Read the model definition and answer for the solid it produces. Units are mm, in the model's axes. Face numbers are marked on the shaded views. Give positions to 0.01 mm unless a question says otherwise; leave off trailing zeros. Order: outer loops, then holes, each group sorted by start corner. A loop starts at its lowest first (then second) coordinate and runs counter-clockwise, first axis right, second up. Notation, with made-up numbers: (-14, -30) - (6, -30) arc R29 ccw to (6, 4) - close; hole circle Ø3 at (-18, 33.25). An arc over 180 degrees is marked (long way). Use a Markdown table: item, result. Add a question column.
1. A cutting plane is placed at B-B on x = 0. Determine the outline of the cut face in (y, z).
2. A cutting plane is placed at D-D on y = -2. Determine the outline of the cut face in (x, z) (1 decimal), and give its area (3 significant figures).
3. A cutting plane is placed at A-A on z = 0. Determine the outline of the cut face in (x, y).
4. Consider L1, parallel to X at y = -2.9, z = 0; L2, parallel to X at y = -4.95, z = 0; L3, parallel to Z at x = 0, y = -5.2. Determine where each line is inside the solid, lowest interval first.
5. A cutting plane is placed at C-C on y = 4. Determine the outline of the cut face in (x, z).
6. For a pull along X with two mould halves and no side action, classify the marked faces 1 and 2 as released by +X, released by -X, zero draft, split by the parting line, or undercut.
7. Flat-ended cylindrical pins translate along their axes: P1, Ø2, axis at y = 8.5, z = -7, coming from the -X side; P2, Ø1.5, axis at y = 10.5, z = -6, coming from the -X side; P3, Ø5, axis at x = 4, z = 0, coming from the +Y side; P4, Ø10, axis at x = -1.5, z = 0.5, coming from the +Y side. Find the tip coordinate at first contact, or state that the pin passes through.
```python
from build123d import *

# Parameters (mm, degrees)
TRUNCATED_BALL_DEPTH      = 13.7
TRUNCATED_BALL_DEPTH_BACK = 13.7
SKETCH8_W                 = 1.5875
SKETCH8_H                 = 11.1125


with BuildPart() as part:
    # Sketch1 → Complete_Ball (revolve)
    with BuildSketch(Plane.XY):
        with BuildLine():
            Line((0, 12.7), (0, -12.7))
            ThreePointArc((0, -12.7), (12.7, 0), (0, 12.7))
        make_face()
    revolve(axis=Axis((0, 13.6525, 0), (0, -1, 0)))

    # Sketch2 → Truncated_ball (cut, two sides)
    with BuildSketch(Plane.XY) as truncated_ball_sk:
        with BuildLine():
            Line((-10.998522628, -6.35), (10.998522628, -6.35))
            ThreePointArc((10.998522628, -6.35), (0, -12.7), (-10.998522628, -6.35))
        make_face()
    extrude(amount=TRUNCATED_BALL_DEPTH, mode=Mode.SUBTRACT)
    extrude(truncated_ball_sk.sketch, amount=-TRUNCATED_BALL_DEPTH_BACK, mode=Mode.SUBTRACT)

    # Sketch8 → Truncated_ball_w_blind_hole (revolve, cut)
    with BuildSketch(Plane.XY):
        with Locations((0.79375, -7.14375)):
            Rectangle(SKETCH8_W, SKETCH8_H)
    revolve(axis=Axis((0, 6.726898043, 0), (0, -1, 0)), mode=Mode.SUBTRACT)


solid = part.part
```
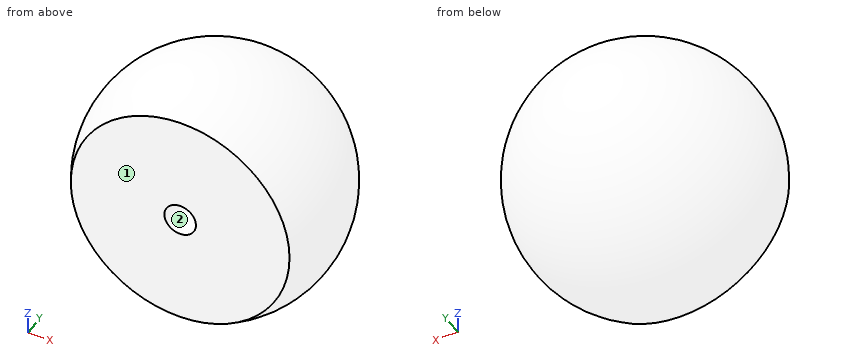
Output values:
| question | item | result |
|---|---|---|
| 1 | outline | (-6.35, -11) arc R12.7 ccw (long way) to (-6.35, 11) - (-6.35, 1.59) - (-1.59, 1.59) - (-1.59, -1.59) - (-6.35, -1.59) - close |
| 2 | outline | circle Ø25.1 at (0, 0); hole circle Ø3.2 at (0, 0) |
| 2 | area | 486 mm² |
| 3 | outline | (-11, -6.35) - (-1.59, -6.35) - (-1.59, -1.59) - (1.59, -1.59) - (1.59, -6.35) - (11, -6.35) arc R12.7 ccw (long way) to start |
| 4 | L1 | -12.36 to -1.59, 1.59 to 12.36 |
| 4 | L2 | -11.7 to -1.59, 1.59 to 11.7 |
| 4 | L3 | -11.59 to -1.59, 1.59 to 11.59 |
| 5 | outline | circle Ø24.11 at (0, 0) |
| 6 | face 1 | zero draft |
| 6 | face 2 | undercut |
| 7 | P1 | x = -7.81 |
| 7 | P2 | x = -5.71 |
| 7 | P3 | y = 12.61 |
| 7 | P4 | y = 12.7 |
